```python
from build123d import *

# Parameters (mm, degrees)
F0_W     = 5
F0_H     = 10
F1_DEPTH = 2.5
F2_W     = 2.5
F2_H     = 6
F3_DEPTH = 7.5
F4_R     = 2.25
F5_DEPTH = 3.44


with BuildPart() as f1:
    # F0 (on Front) → F1 (new body)
    with BuildSketch(Plane.XZ):
        Rectangle(F0_W, F0_H)
    extrude(amount=F1_DEPTH)

    # F2 (on face) → F3 (join)
    with BuildSketch(Plane.XZ.offset(2.5)):
        Rectangle(F2_W, F2_H)
    extrude(amount=F3_DEPTH)

    # F4 (on face) → F5 (cut)
    with BuildSketch(Plane(origin=(-1.25, 0, 0), x_dir=(0, -1, 0), z_dir=(-1, 0, 0))):
        with Locations((6.25, 0)):
            Circle(F4_R)
    extrude(amount=-F5_DEPTH, mode=Mode.SUBTRACT)


solid = f1.part
```
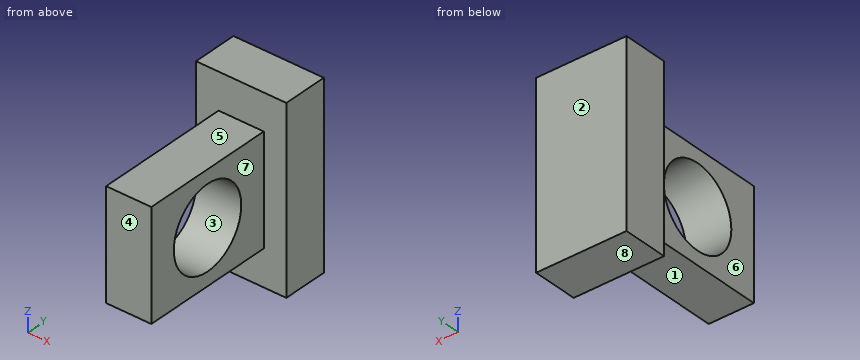
Geometry: final body of the model. Coordinates: model frame, mm. Face numbers are marked on the shaded views. A direction names the side the tool comes from. Coordinates: 2 decimals unless noted, no trailing zeros. Write each loop counter-clockwise with the first axis right and the second up, starting at its lowest first coordinate (ties: lowest second). Pieces come first, ordered by that corner, then holes. Notation, with made-up numbers: M 81,78 L 120,78 A27 cw 120,100 Z; hole C -27,35 d2. An arc over 180 degrees is marked long. Answer as CSV lines item,"result". Start each with the question number.
Q1. Cut plane C-C on z = 2.5. Return the cut outline in (x, y), then the cut area to 4 significant figures.
Q2. Cut plane A-A on y = -6.25. Return the cut outline in (x, z).
Q3. Cut plane D-D on z = -1. Return the cut outline in (x, y), then the cut area to 3 significant figures.
Q4. Cut plane B-B on z = 0. Return the cut outline in (x, y), then the cut area to 3 significant figures.
Q5. Reachability of the marked faces 4, 5, 6, 7 and 8 from +Z, -Z, +X, -X, +Y, -Y: full face, straight path, thin tool, end or side. Return the list, or none.
Q6. Mould query, pull axis Y, two halves, no side actions, for the marked faces 1, 2 and 3. Classes: released by +Y, released by -Y, zero draft, split by the parting line, or undercut.
Q7. Pin query (flat end, axial travel): P1, Ø2, axis at x = 0, y = -5, coming from the -Z side; P2, Ø3, axis at x = 0, y = -7.5, coming from the +Z side; P3, Ø1.8, axis at y = -7.5, z = 1, coming from the +X side; P4, Ø4, axis at y = -6.25, z = 0, coming from the +X side. Return the tip coordinate at first contact, or that it passes through.
Q8. Line query: line 1 (Z direction, x = 0.2, y = -6.25); line 2 (Y direction, x = -1.8, z = 3.25); line 3 (Z direction, x = 0.8, y = -4.25). Output: solid intervals per line, ascending. Write a range as from..to.
Findings below:
1,outline,"M -2.5,-2.5 L -1.25,-2.5 L -1.25,-10 L 1.25,-10 L 1.25,-2.5 L 2.5,-2.5 L 2.5,0 L -2.5,0 Z"
1,area,"31.25 mm2"
2,outline,"M -1.25,-3 L 1.25,-3 L 1.25,-2.25 L -1.25,-2.25 Z; M -1.25,2.25 L 1.25,2.25 L 1.25,3 L -1.25,3 Z"
3,outline,"M -2.5,-2.5 L -1.25,-2.5 L -1.25,-4.23 L 1.25,-4.23 L 1.25,-2.5 L 2.5,-2.5 L 2.5,0 L -2.5,0 Z; M -1.25,-10 L 1.25,-10 L 1.25,-8.27 L -1.25,-8.27 Z"
3,area,"21.2 mm2"
4,outline,"M -2.5,-2.5 L -1.25,-2.5 L -1.25,-4 L 1.25,-4 L 1.25,-2.5 L 2.5,-2.5 L 2.5,0 L -2.5,0 Z; M -1.25,-10 L 1.25,-10 L 1.25,-8.5 L -1.25,-8.5 Z"
4,area,"20.0 mm2"
5,face 4,"+Z, -Z, +X, -X, -Y"
5,face 5,"+Z, +X, -X, -Y"
5,face 6,"+Z, -Z, -X, -Y"
5,face 7,"+Z, -Z, +X, -Y"
5,face 8,"-Z, +X, -X, +Y, -Y"
6,face 1,"zero draft"
6,face 2,"released by +Y"
6,face 3,"undercut"
7,P1,"stops at z = -3"
7,P2,"stops at z = 3"
7,P3,"stops at x = 1.25"
7,P4,"passes through"
8,line 1,"z = -3..-2.25, 2.25..3"
8,line 2,"y = -2.5..0"
8,line 3,"z = -3..-1.03, 1.03..3"
